Could you check a few things on this model? Use its own coordinates, in mm. A direction names the side the tool comes from. Give positions to 0.01 mm unless a question says otherwise; leave off trailing zeros. Order: outer loops, then holes, each group sorted by start corner. A loop starts at its lowest first (then second) coordinate and runs counter-clockwise, first axis right, second up. Notation, with made-up numbers: M 63.5,19 L 76.5,19 A22 ccw 76.5,56 Z; hole C -3,41.5 d1. An arc over 180 degrees is marked long. Use a Markdown table: item, result. Add a question column.
```python
from build123d import *

# Parameters (mm, degrees)
SKETCH1_W           = 7.2
SKETCH1_H           = 3.8
SKETCH1_W_2         = 3.2
SKETCH1_H_2         = 1.25
BOSS_EXTRUDE1_DEPTH = 3
SKETCH6_W           = 13
SKETCH6_H           = 1.25
CUT_EXTRUDE2_DEPTH  = 1.5
BOSS_EXTRUDE2_DEPTH = 3
FILLET1_R           = 1


with BuildPart() as part:
    # Sketch1 → Boss-Extrude1 (new body)
    with BuildSketch(Plane(origin=(0, 0, 0), x_dir=(1, 0, 0), z_dir=(0, 1, 0))):
        Rectangle(SKETCH1_W, SKETCH1_H)
        with Locations((0, 0.16055458)):
            Rectangle(SKETCH1_W_2, SKETCH1_H_2, mode=Mode.SUBTRACT)
    extrude(amount=BOSS_EXTRUDE1_DEPTH)

    # Sketch6 → Cut-Extrude2 (cut)
    with BuildSketch(Plane(origin=(0, 3, 0), x_dir=(1, 0, 0), z_dir=(0, 1, 0))):
        with Locations((1, 0.16055458)):
            Rectangle(SKETCH6_W, SKETCH6_H)
    extrude(amount=-CUT_EXTRUDE2_DEPTH, mode=Mode.SUBTRACT)

    # Sketch7 → Boss-Extrude2 (add)
    with BuildSketch(Plane(origin=(0, 0, -1.9), x_dir=(-1, 0, 0), z_dir=(0, 0, -1))):
        Polygon((-3.6, 0), (3.6, 0), (3.6, 3), (31.4, 3), (31.4, 6.8), (-3.6, 6.8), align=None)
    extrude(amount=BOSS_EXTRUDE2_DEPTH)

    # Fillet1
    fillet1_edges = [part.edges().sort_by_distance(p)[0] for p in [
        (0, 0, -4.9),
    ]]
    fillet(fillet1_edges, radius=FILLET1_R)


solid = part.part
```
1) Suppose I cut it at D-D on z = -3. Please give me the cut outline in (x, y), and give its area (3 significant figures).
2) For faces 5 (the face through (-17, 3, -3)), 6 (the face through (0, 3, 1)), 7 (the face through (-3, 1.5, 0)), 8 (the face through (-1.6, 1, 0)), which set-ups out of +Z, -Z, +X, -X, +Y, -Y let a thin tool reach every point of the face, with its end or its side?
3) Suppose I cut it at B-B on x = -2.5. Please give me the cut outline in (y, z).
4) Please list where these lines run through material, in increasing order: line 1 (Z direction, x = 1.5, y = 2.25); line 2 (X direction, y = 0.5, z = 0.25); line 3 (Y direction, x = -19.5, z = -3.75). Write a range as from..to.
5) Suppose I cut it at C-C on y = 0.5. Please give me the cut outline in (x, z).
6) We'd pull the mould along X, two halves only. Please class faces 1 (the face through (-3.6, 1, -1)), 2 (the face through (0, 2, -0.786)), 3 (the face through (3, 1.5, 0)), 4 (the face through (0, 2, 0.464)): pulls with the +X half, pulls with the -X half, needs draft (parallel to the pull), parting line crosses it, or undercut.
7) Suppose I cut it at A-A on x = 1. Please give me the cut outline in (y, z), and give its area (3 significant figures).
8) For pin 1 (0.6 mm diameter, centred on x = -3, z = 0, fed in from +Y); pin 2 (1 mm diameter, centred on x = -6.5, y = 4.5, fed in from +Z); pin 3 (2 mm diameter, centred on x = -13.5, z = 0, fed in from +Y); pin 4 (3.5 mm diameter, centred on x = -18.5, z = -3, fed in from -Y), each with a flat end and sliding along its axis, tell me the tip position at first contact or that it passes through.
Values found:
| question | item | result |
|---|---|---|
| 1 | outline | M -31.4,3 L -3.6,3 L -3.6,0 L 3.6,0 L 3.6,6.8 L -31.4,6.8 Z |
| 1 | area | 155 mm^2 |
| 2 | face 5 | +Z, -Z, -X, -Y |
| 2 | face 6 | +Z, +X, -X, +Y |
| 2 | face 7 | +X, -X, +Y |
| 2 | face 8 | +Y, -Y |
| 3 | outline | M 0,-3.9 A1 ccw 1,-4.9 L 6.8,-4.9 L 6.8,-1.9 L 3,-1.9 L 3,-0.79 L 1.5,-0.79 L 1.5,0.46 L 3,0.46 L 3,1.9 L 0,1.9 Z |
| 4 | line 1 | z = -4.9..-0.79, 0.46..1.9 |
| 4 | line 2 | x = -3.6..-1.6, 1.6..3.6 |
| 4 | line 3 | y = 3..6.8 |
| 5 | outline | M -3.6,-4.77 L 3.6,-4.77 L 3.6,1.9 L -3.6,1.9 Z; hole M -1.6,-0.79 L 1.6,-0.79 L 1.6,0.46 L -1.6,0.46 Z |
| 6 | face 1 | pulls with the -X half |
| 6 | face 2 | undercut |
| 6 | face 3 | needs draft |
| 6 | face 4 | undercut |
| 7 | outline | M 0,-3.9 A1 ccw 1,-4.9 L 6.8,-4.9 L 6.8,-1.9 L 3,-1.9 L 3,-0.79 L 0,-0.79 Z; M 0,0.46 L 3,0.46 L 3,1.9 L 0,1.9 Z |
| 7 | area | 27.8 mm^2 |
| 8 | pin 1 | stops at y = 1.5 |
| 8 | pin 2 | stops at z = -1.9 |
| 8 | pin 3 | passes through |
| 8 | pin 4 | stops at y = 3 |
